```python
from build123d import *

# Parameters (mm, degrees)
ESQUISSE1_R        = 1.03
ESQUISSE1_W        = 5.9
ESQUISSE1_H        = 7.9
BOSS_EXTRU_1_DEPTH = 6


with BuildPart() as part:
    # Esquisse1 → Boss.-Extru.1 (new body)
    with BuildSketch(Plane.XY):
        Polygon((0, 0), (0, 67.3), (70, 67.3), (70, 6), (65.05, 6), (65.05, 0), (60, 0), (60, 6), (55.05, 6), (55.05, 0), (50, 0), (50, 6), (45.05, 6), (45.05, 0), (40, 0), (40, 6), (35.05, 6), (35.05, 0), (30, 0), (30, 6), (25.05, 6), (25.05, 0), (20, 0), (20, 6), (15.05, 6), (15.05, 0), (10, 0), (10, 6), (5.05, 6), (5.05, 0), align=None)
        with Locations((25, 57.3)):
            Circle(ESQUISSE1_R, mode=Mode.SUBTRACT)
        with Locations((45, 57.3)):
            Circle(ESQUISSE1_R, mode=Mode.SUBTRACT)
        with Locations((25, 37.3)):
            Circle(ESQUISSE1_R, mode=Mode.SUBTRACT)
        with Locations((45, 37.3)):
            Circle(ESQUISSE1_R, mode=Mode.SUBTRACT)
        with Locations((7.5, 59.3)):
            Rectangle(ESQUISSE1_W, ESQUISSE1_H, mode=Mode.SUBTRACT)
        with Locations((62.5, 59.3)):
            Rectangle(ESQUISSE1_W, ESQUISSE1_H, mode=Mode.SUBTRACT)
    extrude(amount=BOSS_EXTRU_1_DEPTH)


solid = part.part
```
Could you check a few things on this model? Use its own coordinates, in mm. A direction names the side the tool comes from. Coordinates: 2 decimals unless noted, no trailing zeros. Write each loop counter-clockwise with the first axis right and the second up, starting at its lowest first coordinate (ties: lowest second). Pieces come first, ordered by that corner, then holes. Notation, with made-up numbers: (60.25, 88) -> (106.25, 88) arc R23 ccw to (106.25, 100) -> close; hole circle Ø4 at (86, -19). An arc over 180 degrees is marked (long way). Write item = value, one per line. Start each with the question number.
(1) I want a section at B-B (x = 9). Please give me the cut outline in (y, z), plus the area to 3 significant figures.
(2) I want a section at C-C (y = 57.3). Please give me the cut outline in (x, z).
(3) I need wall thicknesses on line 1 (Y direction, x = 25, z = 1.6); line 2 (Y direction, x = 7.5, z = 1.75); line 3 (Y direction, x = 62.5, z = 0.95). Which ranges of each line are inside material? Lowest first, please. Write a range as [from, to].
(4) Will these pins go through, and if not, where does the flat tip stop? pin 1 (1 mm diameter, centred on y = 20, z = 3.5, fed in from -X); pin 2 (1.8 mm diameter, centred on y = 1.5, z = 3, fed in from +X); pin 3 (2.5 mm diameter, centred on x = 7, z = 2, fed in from -Y).
(5) I want a section at A-A (y = 37.3). Please give me the cut outline in (x, z), plus the area to 3 significant figures.
(6) We'd pull the mould along X, two halves only. Please class faces 1 (the face through (0, 33, 3)), 2 (the face through (24.87, 38.32, 2.96)), 3 (the face through (35, 34, 6)), 4 (the face through (10, 3, 3)): released by +X, released by -X, zero draft, split by the parting line, or undercut.
(7) I want a section at D-D (z = 3.5). Give the number of separate pieces and of enclosed holes in the cut face, plus the area to 3 significant figures.
(8) Which directions (+Z, -Z, +X, -X, +Y, -Y) give clear straight access to the entire face, cutting with the end or side of a thin tool? Please do faces 5 (the face through (55.05, 3, 3)), 6 (the face through (62, 55.35, 3)).
Result set:
q1.outline = (6, 0) -> (55.35, 0) -> (55.35, 6) -> (6, 6) -> close; (63.25, 0) -> (67.3, 0) -> (67.3, 6) -> (63.25, 6) -> close
q1.area = 320 mm2
q2.outline = (0, 0) -> (4.55, 0) -> (4.55, 6) -> (0, 6) -> close; (10.45, 0) -> (23.97, 0) -> (23.97, 6) -> (10.45, 6) -> close; (26.03, 0) -> (43.97, 0) -> (43.97, 6) -> (26.03, 6) -> close; (46.03, 0) -> (59.55, 0) -> (59.55, 6) -> (46.03, 6) -> close; (65.45, 0) -> (70, 0) -> (70, 6) -> (65.45, 6) -> close
q3.line_1 = [0, 36.27], [38.33, 56.27], [58.33, 67.3]
q3.line_2 = [6, 55.35], [63.25, 67.3]
q3.line_3 = [0, 55.35], [63.25, 67.3]
q4.pin_1 = 0
q4.pin_2 = 65.05
q4.pin_3 = 6
q5.outline = (0, 0) -> (23.97, 0) -> (23.97, 6) -> (0, 6) -> close; (26.03, 0) -> (43.97, 0) -> (43.97, 6) -> (26.03, 6) -> close; (46.03, 0) -> (70, 0) -> (70, 6) -> (46.03, 6) -> close
q5.area = 395 mm2
q6.face_1 = released by -X
q6.face_2 = undercut
q6.face_3 = zero draft
q6.face_4 = undercut
q7.separate_pieces = 1
q7.enclosed_holes = 6
q7.area = 4,400 mm2
q8.face_5 = +Z, -Z, -Y
q8.face_6 = +Z, -Z
